from build123d import *

# Parameters (mm, degrees)
F1_DEPTH = 30
F4_DEPTH = 50
F5_R     = 5
F7_DEPTH = 46


with BuildPart() as f1:
    # F0 (on Front) → F1 (new body)
    with BuildSketch(Plane.XZ):
        Polygon((26.3627171516, 40.0704815984), (-62.9477128386, 36.8853881955), (-46.8072779477, -22.2996752709), (34.61227566, -16.0123351961), align=None)
    extrude(amount=F1_DEPTH)


with BuildPart() as f4:
    # F3 (on Front) → F4 (new body)
    with BuildSketch(Plane.XZ):
        Polygon((101.3598069549, 53.0752539635), (-98.6401930451, 34.245274961), (-112.5807955861, -65.0398209691), (31.4720973372, -49.0130968392), align=None)
    extrude(amount=F4_DEPTH)

    # F5
    f5_edges = [f4.edges().sort_by_distance(p)[0] for p in [
        (101.359807, -25, 53.075254),
    ]]
    fillet(f5_edges, radius=F5_R)

    # F6 (on Front) → F7 (join)
    with BuildSketch(Plane.XZ):
        Polygon((18.8986193389, 48.8469228148), (-44.6650013328, 56.3618317246), (-65.33100456, 2.8180915397), (9.5049822703, -16.9085487723), (42.0695990324, 4.3836981058), align=None)
    extrude(amount=-F7_DEPTH)


solid = f4.part
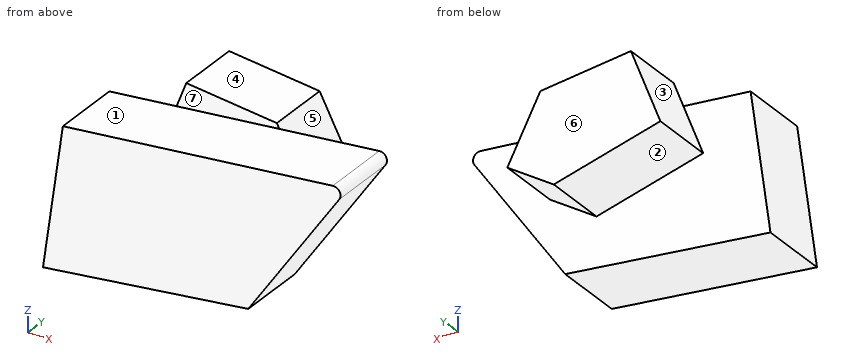
For this review, take the finished solid that the model builds, in its own axes (mm). Face numbers are marked on the shaded views. A direction names the side the tool comes from. Round coordinates to 2 decimals unless told otherwise and drop trailing zeros. Write each loop counter-clockwise with the first axis right and the second up, starting at its lowest first coordinate (ties: lowest second). Pieces come first, ordered by that corner, then holes. Notation, with made-up numbers: (22, -27.5) -> (36, -27.5) arc R35 cw to (36, 4.5) -> close; hole circle Ø2 at (42.25, 83). An arc over 180 degrees is marked (long way). Put each result on its own line as item: value.
Q1. Consider section D-D on y = -35. State the section outline as (x, z) points, and give its area (3 significant figures).
Determined:
outline: (-112.58, -65.04) -> (31.47, -49.01) -> (95.33, 44.27) arc R5 ccw to (90.74, 52.08) -> (-98.64, 34.25) -> close
area: 16,600 mm^2
Q2. To check wall thickness, follow L1, parallel to Y at x = 50.5, z = 47; L2, parallel to Y at x = -24, z = 50; L3, parallel to X at y = 28.5, z = 48.5. State the ranges of each line that lie inside material, in increasing order. Write a range as [from, to].
Determined:
L1: y = [-50, 0]
L2: y = [0, 46]
L3: x = [-47.7, 19.08]
Q3. Machinability: for the marked faces 1, 2, 3 and 4, which of the approach directions +Z, -Z, +X, -X, +Y, -Y give a long, thin tool a straight path to every point of the face, cutting with its end or side? Answer none if there is none.
Determined:
face 1: +Z, -X, -Y
face 2: -Z, -X, +Y
face 3: +Z, -X, +Y
face 4: +Z, +X, +Y, -Y
Q4. Clearance check with flat-ended pins moving along their axes: pin 1 Ø9 at (x, z) = (-20, 47.5) entering from -Y; pin 2 Ø1 at (y, z) = (11, 29) entering from +X; pin 3 Ø12 at (y, z) = (23.5, -3) entering from +X. State where each tip first meets the part, or that it passes through.
Determined:
pin 1: stops at y = 0
pin 2: stops at x = 29.5
pin 3: stops at x = 39.95
Q5. The part is to be moulded in two halves that separate along Y. For the marked faces 5, 6 and 7, say which applies: released by +Y, released by -Y, zero draft, split by the parting line, or undercut.
Determined:
face 5: zero draft
face 6: released by +Y
face 7: released by -Y
Q6. Consider section B-B on z = 13. State the section outline as (x, y) points.
Determined:
outline: (-101.62, -50) -> (73.93, -50) -> (73.93, 0) -> (37.58, 0) -> (37.58, 46) -> (-61.4, 46) -> (-61.4, 0) -> (-101.62, 0) -> close
Q7. Consider section C-C on y = 40. State the section outline as (x, z) points (3 decimals).
Determined:
outline: (-65.331, 2.818) -> (9.505, -16.909) -> (42.07, 4.384) -> (18.899, 48.847) -> (-44.665, 56.362) -> close
Q8. Consider section A-A on x = -59. State the section outline as (y, z) points.
Determined:
outline: (-50, -59.08) -> (0, -59.08) -> (0, 1.15) -> (46, 1.15) -> (46, 19.22) -> (0, 19.22) -> (0, 37.98) -> (-50, 37.98) -> close
